Autodesk Inventor part; units mm, degrees
ref_plane "YZ Plane" through (0, 0, 0) normal (1, 0, 0) x (0, 1, 0)
ref_plane "XZ Plane" through (0, 0, 0) normal (0, 1, 0) x (-1, 0, 0)
ref_plane "XY Plane" through (0, 0, 0) normal (0, 0, 1) x (1, 0, 0)
sketch "Sketch1" plane through (0, 0, 0) normal (0, 0, 1) x (1, 0, 0)
  line L0 (-16.7246, 10.0225) -> (18.2754, 10.0225) construction
  line L1 (53.2754, -19.9775) -> (88.2754, -19.9775) construction
  line L2 (18.2754, 10.0225) -> (53.2754, -19.9775) construction
  line L3 (33.2754, 3.7508) -> (55.125, -14.9775)
  line L4 (55.125, -14.9775) -> (88.2754, -14.9775)
  line L5 (-16.7246, 5.0225) -> (16.4258, 5.0225)
  line L6 (16.4258, 5.0225) -> (51.4258, -24.9775)
  line L7 (51.4258, -24.9775) -> (88.2754, -24.9775)
  line L8 (-21.7246, 10.0225) -> (-21.7246, 10.0225)
  line L9 (93.2754, -19.9775) -> (93.2754, -19.9775)
  arc A0 (-21.7246, 10.0225) -> (-16.7246, 5.0225) centre (-16.7246, 10.0225) ccw
  arc A1 (-16.7246, 15.0225) -> (-21.7246, 10.0225) centre (-16.7246, 10.0225) ccw
  arc A2 (88.2754, -24.9775) -> (93.2754, -19.9775) centre (88.2754, -19.9775) ccw
  arc A3 (93.2754, -19.9775) -> (88.2754, -14.9775) centre (88.2754, -19.9775) ccw
  line L10 (33.2754, 3.7508) -> (33.2754, 25.0225)
  line L11 (23.2754, 35.0225) -> (13.2754, 35.0225)
  line L12 (3.2754, 25.0225) -> (3.2754, 15.0225)
  line L13 (18.2754, 10.0225) -> (18.2754, 35.0225) construction
  line L14 (18.2754, 10.0225) -> (43.2754, 10.0225) construction
  line L15 (3.2754, 25.0225) -> (13.2754, 35.0225)
  line L16 (23.2754, 35.0225) -> (33.2754, 25.0225)
  line L17 (-16.7246, 15.0225) -> (3.2754, 15.0225)
  point P0 (0, 0)
  point P1 (25.9584, 10.0225)
  point P2 (93.2754, -19.9775)
  point P3 (33.2754, 35.0225)
  point P4 (3.2754, 35.0225)
  dimension "d0" = 35
  dimension "d4" = 35
  dimension "d5" = 35
  dimension "d6" = 30
  dimension "d8" = 5
  dimension "d10" = 5
  dimension "d11" = 5
  dimension "d12" = 5
  dimension "d22" = 5
  dimension "d23" = 5
  dimension "d24" = 5
  dimension "d25" = 5
  dimension "d26" = 20
  dimension "d29" = 15
  dimension "d30" = 10
  dimension "d31" = 10
  dimension "d32" = 10
  dimension "d33" = 10
extrude "Extrusion1" add sketch "Sketch1" along normal blind 5
sketch "Sketch2" plane through (0, 0, 5) normal (0, 0, 1) x (1, 0, 0)
  arc A0 (-16.7246, 15.0225) -> (-16.7246, 5.0225) centre (-16.7246, 10.0225) ccw
  arc A1 (88.2754, -24.9775) -> (88.2754, -14.9775) centre (88.2754, -19.9775) ccw
  point P0 (0, 0)
hole "Hole1" at (-16.7246, 10.0225, 5) at (88.2754, -19.9775, 5) direction (0, 0, -1) diameter 5 end through all
sketch "Sketch3" plane through (0, 0, 5) normal (0, 0, 1) x (1, 0, 0)
  circle A0 centre (18.2559, 19.7273) radius 12.5 construction
  point P0 (0, 0)
  dimension "d34" = 25
properties part number "BrazoTV2" material "MDF Medium Density Fiberboard"
Can you work these out from the model? Positions are in its coordinate system, mm. A direction names the side the tool comes from. Round coordinates to 2 decimals unless told otherwise and drop trailing zeros. Loops run counter-clockwise (first coordinate to the right, second up) from the corner with the lowest first, then second, coordinate; pieces in that order, holes last. Notation, with made-up numbers: M -40,-13 L 17,-13 A22 cw 17,17 Z; hole C -5,49.25 d2. An arc over 180 degrees is marked long. Answer in a Markdown table with one row per item.
1. I'm going to push flat-ended pins straight in: pin 1 Ø2.5 at (x, z) = (-7, 2.5) entering from +Y; pin 2 Ø2.5 at (y, z) = (21, 3) entering from -X; pin 3 Ø3 at (y, z) = (-18.5, 2) entering from -X; pin 4 Ø6 at (x, y) = (88.28, -19.98) entering from +Z. Where does each tip first touch, or does it pass through?
Established:
| item | result |
|---|---|
| pin 1 | y = 15.02 |
| pin 2 | x = 3.28 |
| pin 3 | x = 42.12 |
| pin 4 | z = 5 |
2. On a 3-axis mill with a long thin cutter (end or side, diameter ignored), from which of +Z, -Z, +X, -X, +Y, -Y can I reach the whole of each face in a straight line? I mean faces 4 (the face through (33.275, 14, 2)), 5 (the face through (27, 3, 5)), 6 (the face through (18, 35.022, 2)), 7 (the face through (-7, 15.022, 2)), 8 (the face through (0, 5.022, 2)). Say none if no direction works.
Established:
| item | result |
|---|---|
| face 4 | +Z, -Z, +X, +Y |
| face 5 | +Z, +X, -X, +Y, -Y |
| face 6 | +Z, -Z, +X, -X, +Y |
| face 7 | +Z, -Z, -X, +Y |
| face 8 | +Z, -Z, -X, -Y |
3. Thinking about a two-plate mould opening in Y: for faces 1 (the face through (27, 3, 0)), 2 (the face through (85.797, -19.652, 2.465)), 3 (the face through (70, -24.978, 2)), which applies, pulls with the +Y half, pulls with the -Y half, needs draft (parallel to the pull), parting line crosses it, or undercut?
Established:
| item | result |
|---|---|
| face 1 | needs draft |
| face 2 | undercut |
| face 3 | pulls with the -Y half |
4. If we section it at B-B, the plane y = 10.5: Please give me the cut outline in (x, z), plus the area to 3 significant figures.
Established:
| item | result |
|---|---|
| outline | M -21.7,0 L -19.18,0 L -19.18,5 L -21.7,5 Z; M -14.27,0 L 33.28,0 L 33.28,5 L -14.27,5 Z |
| area | 250 mm² |
5. If we section it at A-A, the plane z = 1.4: Please give me the cut outline in (x, y) (1 decimal).
Established:
| item | result |
|---|---|
| outline | M -16.7,5 L 16.4,5 L 51.4,-25 L 88.3,-25 A5 ccw 88.3,-15 L 55.1,-15 L 33.3,3.8 L 33.3,25 L 23.3,35 L 13.3,35 L 3.3,25 L 3.3,15 L -16.7,15 A5 ccw Z; hole C -16.7,10 d5; hole C 88.3,-20 d5 |
6. If we section it at D-D, the plane y = -2: Please give me the cut outline in (x, z).
Established:
| item | result |
|---|---|
| outline | M 24.62,0 L 39.98,0 L 39.98,5 L 24.62,5 Z |
7. Please list where these lines run through material, in increasing order: line 1 (Y direction, x = 73, z = 0.6); line 2 (Y direction, x = -14.5, z = 0.4); line 3 (X direction, y = 23, z = 0.3). Write a range as from..to.
Established:
| item | result |
|---|---|
| line 1 | -24.98..-14.98 |
| line 2 | 5.02..8.88, 11.16..15.02 |
| line 3 | 3.28..33.28 |
8. If we section it at C-C, the plane x = 69: Please give me the cut outline in (y, z).
Established:
| item | result |
|---|---|
| outline | M -24.98,0 L -14.98,0 L -14.98,5 L -24.98,5 Z |
